```python
from build123d import *

# Parameters (mm, degrees)
SKETCH1_R               = 5
BOSS_EXTRUDE1_DEPTH     = 19
CUT_EXTRUDE1_DEPTH      = 21.273134933
CUT_EXTRUDE1_DEPTH_BACK = 21.273134933
SKETCH3_R               = 1.75
CUT_EXTRUDE2_DEPTH      = 20
SKETCH4_R               = 1.25
CUT_EXTRUDE3_DEPTH      = 21.273135076


with BuildPart() as part:
    # Sketch1 → Boss-Extrude1 (new, symmetric)
    with BuildSketch(Plane(origin=(0, 0, 0), x_dir=(0, 0, -1), z_dir=(1, 0, 0))):
        Circle(SKETCH1_R)
    extrude(amount=BOSS_EXTRUDE1_DEPTH, both=True)

    # Sketch2 → Cut-Extrude1 (cut, two sides: drawn at the far end of the back side and taken through both)
    with BuildSketch(Plane.XY.offset(-CUT_EXTRUDE1_DEPTH_BACK)):
        with BuildLine():
            Line((-67.696223967, 62.386645779), (-13.856406461, 5))
            ThreePointArc((-13.856406461, 5), (0, -1), (13.856406461, 5))
            Line((13.856406461, 5), (67.696223967, 62.386645779))
            Line((67.696223967, 62.386645779), (67.696223967, 219.764573876))
            Line((67.696223967, 219.764573876), (-67.696223967, 219.764573876))
            Line((-67.696223967, 219.764573876), (-67.696223967, 62.386645779))
        make_face()
    extrude(amount=CUT_EXTRUDE1_DEPTH + CUT_EXTRUDE1_DEPTH_BACK, mode=Mode.SUBTRACT)

    # Sketch3 → Cut-Extrude2 (cut, symmetric)
    with BuildSketch(Plane(origin=(0, 0, 0), x_dir=(0, 0, -1), z_dir=(1, 0, 0))):
        Circle(SKETCH3_R)
    extrude(amount=CUT_EXTRUDE2_DEPTH, both=True, mode=Mode.SUBTRACT)

    # Sketch4 → Cut-Extrude3 (cut, through all)
    with BuildSketch(Plane(origin=(0, 0, 0), x_dir=(1, 0, 0), z_dir=(0, 1, 0))):
        with Locations(Location((0, 0, 0), (0, 0, 270))):
            Circle(SKETCH4_R)
    extrude(amount=-CUT_EXTRUDE3_DEPTH, mode=Mode.SUBTRACT)


solid = part.part
```
Verification items for the finished model (mm, model axes). Coordinates: 2 decimals unless noted, no trailing zeros. Write each loop counter-clockwise with the first axis right and the second up, starting at its lowest first coordinate (ties: lowest second). Pieces come first, ordered by that corner, then holes. Notation, with made-up numbers: M 43.25,-33 L 87.25,-33 A16 ccw 87.25,-16 Z; hole C 44,78 d1. An arc over 180 degrees is marked long. One line per item, written item: value.
Item 1: Gauge pin test, flat ends, axial feed: pin 1 Ø1.5 at (x, z) = (-11, -2.5) entering from -Y; pin 2 Ø4 at (x, y) = (11, -2) entering from +Z; pin 3 Ø4 at (x, z) = (0, 0) entering from +Y; pin 4 Ø1.5 at (x, y) = (13.5, -3) entering from +Z. Record the tip position at first contact, or that the pin passes through.
Check sheet entries:
pin 1: stops at y = -4.68
pin 2: stops at z = 5
pin 3: stops at y = -0.95
pin 4: stops at z = 4.47
Item 2: Section check D-D, the plane y = 0. Record the boundary of the cut face in (x, z).
Check sheet entries:
outline: M -19,-5 L -6.08,-5 L -6.08,-1.75 L -19,-1.75 Z; M -19,1.75 L -6.08,1.75 L -6.08,5 L -19,5 Z; M 6.08,-5 L 19,-5 L 19,-1.75 L 6.08,-1.75 Z; M 6.08,1.75 L 19,1.75 L 19,5 L 6.08,5 Z
Item 3: Section check B-B, the plane z = 0. Record the boundary of the cut face in (x, y).
Check sheet entries:
outline: M -19,-5 L -1.25,-5 L -1.25,-1.75 L -19,-1.75 Z; M -19,1.75 L -9.85,1.75 A19 cw -13.86,5 L -19,5 Z; M 1.25,-5 L 19,-5 L 19,-1.75 L 1.25,-1.75 Z; M 9.85,1.75 L 19,1.75 L 19,5 L 13.86,5 A19 cw Z
Item 4: Section check C-C, the plane x = 14.5. Record the boundary of the cut face in (y, z), plus the area to 3 significant figures.
Check sheet entries:
outline: C 0,0 d10; hole C 0,0 d3.5
area: 68.9 mm^2
Item 5: Mould release check, pull along Y, two halves, no side actions. Record for faces 1 (the cylindrical face through (4.49, -1.71, 0.38)), 2 (the cylindrical face through (0.38, -3.09, 1.19)), 3 (the cylindrical face through (0, -1, 2)): pulls with the +Y half, pulls with the -Y half, needs draft (parallel to the pull), parting line crosses it, or undercut.
Check sheet entries:
face 1: undercut
face 2: needs draft
face 3: pulls with the +Y half
Item 6: Scan lines: line 1 along X through (y, z) = (-3, 0); line 2 along Z through (x, y) = (-6.5, 0); line 3 along X through (y, z) = (-4.5, 1). Record each from-to range of solid material in increasing order.
Check sheet entries:
line 1: x = -19 to -1.25, 1.25 to 19
line 2: z = -5 to -1.75, 1.75 to 5
line 3: x = -19 to -0.75, 0.75 to 19
Item 7: Section check A-A, the plane y = 2.5. Record the boundary of the cut face in (x, z), plus the area to 3 significant figures.
Check sheet entries:
outline: M -19,-4.33 L -10.99,-4.33 L -10.99,4.33 L -19,4.33 Z; M 10.99,-4.33 L 19,-4.33 L 19,4.33 L 10.99,4.33 Z
area: 139 mm^2
